Build history of the part. All positions in model axes, mm. A direction names the side the tool comes from. Coordinates: 2 decimals unless noted, no trailing zeros. Loops run counter-clockwise (first coordinate to the right, second up) from the corner with the lowest first, then second, coordinate; pieces in that order, holes last.
(1) Wall check: L1, parallel to X at y = -22, z = -13; L2, parallel to Y at x = -34.75, z = 7.5; L3, parallel to Z at x = -52, y = -50. Give the ranges that are in metal, low to high.
(2) Slice it at A-A (y = -50.5). Give the cut face in (x, z), and give its area (3 significant figures).
(3) Slice it at B-B (x = -35). Give the cut face in (y, z), and give its area (3 significant figures).
(4) Flat gauge pins, fed straight in: P1, Ø8, axis at x = -39.5, y = -52.5, coming from the +Z side; P2, Ø7, axis at y = -46.5, z = 6.5, coming from the -X side; P3, Ø3, axis at x = 62.5, y = 2.5, coming from the +Z side. Where does each tip first touch, or does it go through?
(5) Tool access for faces 5 (the face through (-37, -49, 15)), 6 (the face through (-55, -58, 0)), 7 (the face through (-60, -34, 0)), 8 (the face through (64.93, -2.993, -9.542)), 9 (the face through (-55, 1, -34)): list every direction of +Z, -Z, +X, -X, +Y, -Y with a clear straight run to the whole face (end or side of a thin tool).
(6) Slice it at D-D (z = 22.5). Give the cut face in (x, y), and give its area (3 significant figures).
(7) Slice it at C-C (y = 16). Give the cut face in (x, z), and give its area (3 significant figures).
(8) Two-plate mould, pull along Z, no slides. Class faces 1 (the face through (-37.07, -47.97, 9.11)), 2 (the face through (-37, -49, -15)), 3 (the face through (50, 1, -34)), 4 (the face through (58, -35, 0)): pulls with the +Z half, pulls with the -Z half, needs draft (parallel to the pull), parting line crosses it, or undercut.
from build123d import *

# Parameters (mm, degrees)
BOSS_EXTRUDE1_DEPTH      = 60
BOSS_EXTRUDE2_START      = -5
BOSS_EXTRUDE2_DEPTH      = 5
BOSS_EXTRUDE3_START      = 10
BOSS_EXTRUDE3_DEPTH      = 10
BOSS_EXTRUDE4_DEPTH      = 15
BOSS_EXTRUDE4_2_DEPTH    = 15
BOSS_EXTRUDE6_REACH      = 104.54
BOSS_EXTRUDE6_END_RADIUS = 43
SKETCH5_W                = 10
SKETCH5_H                = 30
CUT_EXTRUDE1_REACH       = 147.592
SKETCH6_R                = 3
SKETCH7_R                = 35
CUT_EXTRUDE2_DEPTH       = 5
LPATTERN1_COUNT          = 2
LPATTERN1_PITCH          = 110
FILLET1_R                = 2
CUT_EXTRUDE3_REACH       = 140.611


with BuildPart() as part:
    # Sketch1 → Boss-Extrude1 (new, symmetric)
    with BuildSketch(Plane(origin=(0, 0, 0), x_dir=(0, 0, -1), z_dir=(1, 0, 0))):
        with BuildLine():
            Line((-38.065732621, -20), (-26.248809497, -20))
            ThreePointArc((-26.248809497, -20), (0, -33), (26.248809497, -20))
            Line((26.248809497, -20), (38.065732621, -20))
            ThreePointArc((38.065732621, -20), (0, -43), (-38.065732621, -20))
        make_face()
    extrude(amount=BOSS_EXTRUDE1_DEPTH, both=True)

    # Sketch2 → Boss-Extrude2 (add)
    with BuildSketch(Plane(origin=(60, 0, 0), x_dir=(0, 0, -1), z_dir=(1, 0, 0)).offset(BOSS_EXTRUDE2_START)):
        with BuildLine():
            Line((-31.304951685, 21.540659229), (-25, 21.540659229))
            ThreePointArc((-25, 21.540659229), (0, -33), (25, 21.540659229))
            Line((25, 21.540659229), (31.304951685, 21.540659229))
            ThreePointArc((31.304951685, 21.540659229), (0, -38), (-31.304951685, 21.540659229))
        make_face()
    boss_extrude2 = extrude(amount=-BOSS_EXTRUDE2_DEPTH)

    # Sketch3 → Boss-Extrude3 (add)
    with BuildSketch(Plane(origin=(60, 0, 0), x_dir=(0, 0, -1), z_dir=(1, 0, 0)).offset(BOSS_EXTRUDE3_START)):
        with BuildLine():
            Line((-26.248809497, -20), (-26.248809497, 21.540659229))
            Line((-26.248809497, 21.540659229), (26.248809497, 21.540659229))
            Line((26.248809497, 21.540659229), (26.248809497, -20))
            Line((26.248809497, -20), (38.065732621, -20))
            ThreePointArc((38.065732621, -20), (0, -43), (-38.065732621, -20))
            Line((-38.065732621, -20), (-26.248809497, -20))
        make_face()
    extrude(amount=-BOSS_EXTRUDE3_DEPTH)



with BuildPart() as body_2:
    # Sketch4 → Boss-Extrude4 (new, symmetric)
    with BuildSketch(Plane.XY):
        with BuildLine():
            Line((-48, -43), (-48, -54))
            ThreePointArc((-48, -54), (-49.171572875, -56.828427125), (-52, -58))
            Line((-52, -58), (-58, -58))
            Line((-58, -58), (-58, -43))
            Line((-58, -43), (-48, -43))
        make_face()
    extrude(amount=BOSS_EXTRUDE4_DEPTH, both=True)


with BuildPart() as body_3:
    # Sketch4 → Boss-Extrude4 2 (new, symmetric)
    with BuildSketch(Plane.XY):
        with BuildLine():
            Line((-32, -43), (-42, -43))
            Line((-42, -43), (-42, -54))
            ThreePointArc((-42, -54), (-40.828427125, -56.828427125), (-38, -58))
            Line((-38, -58), (-32, -58))
            Line((-32, -58), (-32, -43))
        make_face()
    extrude(amount=BOSS_EXTRUDE4_2_DEPTH, both=True)


with BuildPart() as part_1:
    add(part.part)

    add(body_2.part)  # Boss-Extrude6 merges body 2

    add(body_3.part)  # Boss-Extrude6 merges body 3
    # Boss-Extrude6: up to this cylinder (the profile starts outside it)
    boss_extrude6_end = Plane(origin=(-45, 0, 0), z_dir=(-1, 0, 0)) * Cylinder(BOSS_EXTRUDE6_END_RADIUS, 312.08, mode=Mode.PRIVATE)
    # Sketch5 → Boss-Extrude6 (add, up to the surface)
    with BuildSketch(Plane(origin=(0, -43, 0), x_dir=(1, 0, 0), z_dir=(0, 1, 0)), mode=Mode.PRIVATE) as boss_extrude6_sk1:
        with Locations((-37, 0)):
            Rectangle(SKETCH5_W, SKETCH5_H)
    boss_extrude6_tool1 = extrude(boss_extrude6_sk1.sketch, amount=BOSS_EXTRUDE6_REACH, mode=Mode.PRIVATE) - boss_extrude6_end
    add(boss_extrude6_tool1.solids().sort_by_distance((-37, -43, 0))[0])
    add(boss_extrude6_tool1.solids().sort_by_distance((-37, -43, 0))[1])
    # Sketch5 → Boss-Extrude6 (add, up to the surface)
    with BuildSketch(Plane(origin=(0, -43, 0), x_dir=(1, 0, 0), z_dir=(0, 1, 0)), mode=Mode.PRIVATE) as boss_extrude6_sk2:
        with Locations((-53, 0)):
            Rectangle(SKETCH5_W, SKETCH5_H)
    boss_extrude6_tool2 = extrude(boss_extrude6_sk2.sketch, amount=BOSS_EXTRUDE6_REACH, mode=Mode.PRIVATE) - boss_extrude6_end
    add(boss_extrude6_tool2.solids().sort_by_distance((-53, -43, 0))[0])
    add(boss_extrude6_tool2.solids().sort_by_distance((-53, -43, 0))[1])

    # Cut-Extrude1: up to this face of the body (flat: up to its plane)
    cut_extrude1_end = Plane(part_1.part.faces().sort_by_distance((-32, -50.035411039, 0))[0])
    # Sketch6 → Cut-Extrude1 (cut, up to the picked face)
    with BuildSketch(Plane.ZY.offset(58), mode=Mode.PRIVATE) as cut_extrude1_sk1:
        with Locations((-7.5, -50.5)):
            Circle(SKETCH6_R)
    cut_extrude1_tool1 = split(extrude(cut_extrude1_sk1.sketch, amount=-CUT_EXTRUDE1_REACH, mode=Mode.PRIVATE), bisect_by=cut_extrude1_end, keep=Keep.BOTH, mode=Mode.PRIVATE)
    # Sketch6 → Cut-Extrude1 (cut, up to the picked face)
    with BuildSketch(Plane.ZY.offset(58), mode=Mode.PRIVATE) as cut_extrude1_sk2:
        with Locations((7.5, -50.5)):
            Circle(SKETCH6_R)
    cut_extrude1_tool2 = split(extrude(cut_extrude1_sk2.sketch, amount=-CUT_EXTRUDE1_REACH, mode=Mode.PRIVATE), bisect_by=cut_extrude1_end, keep=Keep.BOTH, mode=Mode.PRIVATE)
    add(cut_extrude1_tool1.solids().sort_by(Axis((-58, -50.5, -7.5), (1, 0, 0)))[0], mode=Mode.SUBTRACT)
    add(cut_extrude1_tool2.solids().sort_by(Axis((-58, -50.5, 7.5), (1, 0, 0)))[0], mode=Mode.SUBTRACT)

    # Sketch7 → Cut-Extrude2 (cut)
    with BuildSketch(Plane.ZY.offset(-60)):
        Circle(SKETCH7_R)
    extrude(amount=CUT_EXTRUDE2_DEPTH, mode=Mode.SUBTRACT)

    # LPattern1: Boss-Extrude2 ×2
    with Locations(*[(-i * LPATTERN1_PITCH, 0, 0) for i in range(1, LPATTERN1_COUNT)]):
        add(boss_extrude2)

    # Fillet1
    fillet1_edges = [part_1.edges().sort_by_distance(p)[0] for p in [
        (52.5, 21.540659229, 25),
        (52.5, 21.540659229, -31.304951685),
        (52.5, 21.540659229, -25),
        (-57.5, 21.540659229, 25),
        (-57.5, 21.540659229, -31.304951685),
        (-57.5, 21.540659229, -25),
        (-57.5, 21.540659229, 31.304951685),
        (52.5, 21.540659229, 31.304951685),
    ]]
    fillet(fillet1_edges, radius=FILLET1_R)

    # Sketch8 → Cut-Extrude3 (cut, up to next)
    with BuildSketch(Plane.ZY.offset(-60), mode=Mode.PRIVATE) as cut_extrude3_sk1:
        Polygon((0, 12.360679775), (-11.755705046, 3.819660113), (-7.26542528, -10), (7.26542528, -10), (11.755705046, 3.819660113), align=None)
    cut_extrude3_tool1 = extrude(cut_extrude3_sk1.sketch, amount=-CUT_EXTRUDE3_REACH, mode=Mode.PRIVATE) & part_1.part
    add(cut_extrude3_tool1.solids().sort_by_distance((60, 0, 0))[0], mode=Mode.SUBTRACT)


solid = part_1.part
Response values:
1. L1: x = 60 to 70
1. L2: y = -58 to -53.5, -47.5 to -32.14
1. L3: z = -15 to -10.46, -4.54 to 4.54, 10.46 to 15
2. outline: (-58, -15) - (-48, -15) - (-48, -10.5) - (-58, -10.5) - close; (-58, -4.5) - (-48, -4.5) - (-48, 4.5) - (-58, 4.5) - close; (-58, 10.5) - (-48, 10.5) - (-48, 15) - (-58, 15) - close; (-42, -15) - (-32, -15) - (-32, -10.5) - (-42, -10.5) - close; (-42, -4.5) - (-32, -4.5) - (-32, 4.5) - (-42, 4.5) - close; (-42, 10.5) - (-32, 10.5) - (-32, 15) - (-42, 15) - close
2. area: 360 mm2
3. outline: (-58, -15) - (-40.3, -15) arc R43 ccw to (-20, -38.07) - (-20, -26.25) arc R33 cw to (-20, 26.25) - (-20, 38.07) arc R43 ccw to (-40.3, 15) - (-58, 15) - close; hole circle Ø6 at (-50.5, -7.5); hole circle Ø6 at (-50.5, 7.5)
3. area: 1,190 mm2
4. P1: stops at z = 15
4. P2: stops at x = -58
4. P3: stops at z = 26.25
5. face 5: +Z, +X, -X, -Y
5. face 6: +Z, -Z, +X, -X, -Y
5. face 7: +Z, -Z, -X, +Y, -Y
5. face 8: +X, -X
5. face 9: +Z, -Z, +Y
6. outline: (-60, -36.64) - (70, -36.64) - (70, 21.54) - (60, 21.54) - (60, -26.81) - (55, -26.81) - (55, -24.14) - (-60, -24.14) - close
6. area: 2,070 mm2
7. outline: (-60, -34.47) - (-55, -34.47) - (-55, -28.86) - (-60, -28.86) - close; (-60, 28.86) - (-55, 28.86) - (-55, 34.47) - (-60, 34.47) - close; (50, -34.47) - (55, -34.47) - (55, -28.86) - (50, -28.86) - close; (50, 28.86) - (55, 28.86) - (55, 34.47) - (50, 34.47) - close; (60, -26.25) - (70, -26.25) - (70, 26.25) - (60, 26.25) - close
7. area: 637 mm2
8. face 1: undercut
8. face 2: pulls with the -Z half
8. face 3: needs draft
8. face 4: undercut
